from build123d import *

# Parameters (mm, degrees)
F1_DEPTH = 304.8
F3_DEPTH = 50.8
F4_D     = 12.7


with BuildPart() as f1:
    # F0 (on Top) → F1 (new body)
    with BuildSketch(Plane.XY):
        with BuildLine():
            Line((-12.7, -44.45), (12.7, -44.45))
            ThreePointArc((12.7, -44.45), (17.1901280605, -42.5901280605), (19.05, -38.1))
            Line((19.05, -38.1), (19.05, 38.1))
            ThreePointArc((19.05, 38.1), (17.1901280605, 42.5901280605), (12.7, 44.45))
            Line((12.7, 44.45), (-12.7, 44.45))
            ThreePointArc((-12.7, 44.45), (-17.1901280605, 42.5901280605), (-19.05, 38.1))
            Line((-19.05, 38.1), (-19.05, -38.1))
            ThreePointArc((-19.05, -38.1), (-17.1901280605, -42.5901280605), (-12.7, -44.45))
        make_face()
    extrude(amount=F1_DEPTH)

    # F2 (on face) → F3 (cut)
    with BuildSketch(Plane(origin=(-19.05, 0, 0), x_dir=(0, -1, 0), z_dir=(-1, 0, 0))):
        Polygon((-38.1, 304.8), (-44.45, 304.8), (-44.45, 278.7617928475), (-38.1, 285.1117928475), align=None)
        Polygon((-18.4117928475, 304.8), (-38.1, 304.8), (-38.1, 285.1117928475), align=None)
        Polygon((-38.1, 19.6882071525), (-44.45, 26.0382071525), (-44.45, 0), (-38.1, 0), align=None)
        Polygon((-18.4117928475, 0), (-38.1, 19.6882071525), (-38.1, 0), align=None)
        Polygon((38.1, 304.8), (18.4117928475, 304.8), (38.1, 285.1117928475), align=None)
        Polygon((44.45, 304.8), (38.1, 304.8), (38.1, 285.1117928475), (44.45, 278.7617928475), align=None)
        Polygon((38.1, 19.6882071525), (18.4117928475, 0), (38.1, 0), align=None)
        Polygon((44.45, 26.0382071525), (38.1, 19.6882071525), (38.1, 0), (44.45, 0), align=None)
    extrude(amount=-F3_DEPTH, mode=Mode.SUBTRACT)

    # F4 (through all)
    with Locations(Plane(origin=(-19.05, 0, 0), x_dir=(0, -1, 0), z_dir=(-1, 0, 0))):
        with Locations((0, 76.2), (0, 228.6)):
            Hole(F4_D / 2)


solid = f1.part
Check sheet for the modelled part. Datum: model origin and axes. Units: mm. Give positions to 0.01 mm unless a question says otherwise; leave off trailing zeros. Order: outer loops, then holes, each group sorted by start corner. A loop starts at its lowest first (then second) coordinate and runs counter-clockwise, first axis right, second up. Notation, with made-up numbers: M -32.5,55 L 3.5,55 A33 ccw 3.5,86 Z; hole C 51.25,72 d10. An arc over 180 degrees is marked long. Answer as CSV lines item,"result". Start each with the question number.
Item 1: Cross-section at A-A on z = 76.2. Enter the section's corners in (x, y), plus the area to 3 significant figures.
Item 2: Cross-section at B-B on y = 0. Enter the section's corners in (x, z).
Item 3: Cross-section at D-D on y = 21. Enter the section's corners in (x, z), plus the area to 3 significant figures.
Item 4: Thickness scan on line 1 (Z direction, x = 11, y = 0); line 2 (Y direction, x = 0, z = 76); line 3 (Z direction, x = -11, y = -4.5). Record the ranges inside material, lowest first. Write a range as [from, to].
Item 5: Cross-section at C-C on x = 2. Enter the section's corners in (y, z), plus the area to 3 significant figures.
Item 6: Mould release check, pull along Y, two halves, no side actions. Record for faces 1 (the face through (0.27, -1.38, 222.4)), 2 (the face through (17.14, -42.64, 150.54)), 3 (the face through (0, 44.45, 151)), 4 (the face through (0.27, -1.38, 70)): +Y half, -Y half, draft (parallel to the pull), parting line (faces both ways), or undercut.
Item 7: Gauge pin test, flat end, axial feed: P1, Ø10, axis at x = 2, y = 24.5, coming from the -Z side. Record the tip position at first contact, or that the pin passes through.
Established:
1,outline,"M -19.05,-38.1 A6.35 ccw -12.7,-44.45 L 12.7,-44.45 A6.35 ccw 19.05,-38.1 L 19.05,-6.35 L -19.05,-6.35 Z; M -19.05,6.35 L 19.05,6.35 L 19.05,38.1 A6.35 ccw 12.7,44.45 L -12.7,44.45 A6.35 ccw -19.05,38.1 Z"
1,area,"2,870 mm^2"
2,outline,"M -19.05,0 L 19.05,0 L 19.05,69.85 L -19.05,69.85 Z; M -19.05,82.55 L 19.05,82.55 L 19.05,222.25 L -19.05,222.25 Z; M -19.05,234.95 L 19.05,234.95 L 19.05,304.8 L -19.05,304.8 Z"
3,outline,"M -19.05,2.59 L 19.05,2.59 L 19.05,302.21 L -19.05,302.21 Z"
3,area,"11,400 mm^2"
4,line 1,"z = [0, 69.85], [82.55, 222.25], [234.95, 304.8]"
4,line 2,"y = [-44.45, -6.35], [6.35, 44.45]"
4,line 3,"z = [0, 71.72], [80.68, 224.12], [233.08, 304.8]"
5,outline,"M -44.45,26.04 L -18.41,0 L 18.41,0 L 44.45,26.04 L 44.45,278.76 L 18.41,304.8 L -18.41,304.8 L -44.45,278.76 Z; hole C 0,76.2 d12.7; hole C 0,228.6 d12.7"
5,area,"25,500 mm^2"
6,face 1,"undercut"
6,face 2,"-Y half"
6,face 3,"+Y half"
6,face 4,"undercut"
7,P1,"stops at z = 1.09"
